The model under review builds one solid part; all positions refer to its coordinate system, in mm. A direction names the side the tool comes from. Give positions to 0.01 mm unless a question says otherwise; leave off trailing zeros. Order: outer loops, then holes, each group sorted by start corner. A loop starts at its lowest first (then second) coordinate and runs counter-clockwise, first axis right, second up. Notation, with made-up numbers: (-12, 72.5) -> (38, 72.5) arc R8 cw to (38, 79.5) -> close; hole circle Ø9 at (26.5, 88.5). An arc over 180 degrees is marked (long way). Answer as a JSON object with one key per item and string values. Group by question number.
from build123d import *

# Parameters (mm, degrees)
F0_R     = 3.5
F0_R_2   = 3
F1_DEPTH = 17.016
F3_R     = 4.5
F3_R_2   = 3.5
F4_DEPTH = 16
F6_W     = 16
F6_H     = 9


with BuildPart() as f1:
    # F0 (on Top) → F1 (new body)
    with BuildSketch(Plane.XY):
        Circle(F0_R)
        Circle(F0_R_2, mode=Mode.SUBTRACT)
    extrude(amount=F1_DEPTH)

    # F3 (on offset) → F4 (join, through all)
    with BuildSketch(Plane.XY.offset(1.016)):
        Circle(F3_R)
        Circle(F3_R_2, mode=Mode.SUBTRACT)
    extrude(amount=F4_DEPTH)

    # F6 (on offset) → F7 section 0
    with BuildSketch(Plane.XY.offset(17.016), mode=Mode.PRIVATE) as f7_s0:
        Rectangle(F6_W, F6_H)
    loft([f7_s0.sketch, Vertex(0, 0, 1.016)], mode=Mode.SUBTRACT)


solid = f1.part
1. Take a section at A-A on x = 0. Give the boundary of the cut face in (y, z).
2. For probe 1 along Y at (x, z) = (0, 3.5); probe 2 along X at (y, z) = (0, 8.75), list the stretches that pass through material, from the lowest coordinate up. Write a range as [from, to].
3. For pin 1 (1.5 mm diameter, centred on x = -2, z = 14.5, fed in from +Y); pin 2 (2 mm diameter, centred on x = -1.5, z = 10.5, fed in from +Y); pin 3 (4 mm diameter, centred on y = -3.5, z = 6.5, fed in from -X), all flat-tipped, find the tip position at first contact; note any pin that passes through.
4. Take a section at D-D on x = 3.25. Give the boundary of the cut face in (y, z), plus the area to 3 significant figures.
5. Take a section at C-C on z = 10.25. Give the boundary of the cut face in (x, y).
6. Machinability: for faces 1 (the flat face through (3, 1, 0)), 2 (the flat face through (3.54, -0.03, 8.1)), 3 (the cylindrical face through (3.233, -1.341, 0.501)), which of the approach directions +Z, -Z, +X, -X, +Y, -Y give a long, thin tool a straight path to every point of the face, cutting with its end or side? Answer none if there is none.
7. Take a section at B-B on y = 0. Give the boundary of the cut face in (x, z).
8. Draft analysis for pull direction X (two halves, no side actions). For faces 4 (the cylindrical face through (4.292, 1.352, 7.126)), 5 (the cylindrical face through (2.86, 0.9, 4.48)), 6 (the flat face through (0, -4, 1.016)), state which applies: pulls with the +X half, pulls with the -X half, needs draft (parallel to the pull), parting line crosses it, or undercut.
Checks:
{
 "1": {"outline": "(-4.5, 1.02) -> (-3.5, 1.02) -> (-3.5, 0) -> (-3, 0) -> (-3, 11.68) -> (-4.5, 17.02) -> close; (3, 0) -> (3.5, 0) -> (3.5, 1.02) -> (4.5, 1.02) -> (4.5, 17.02) -> (3, 11.68) -> close"},
 "2": {"probe 1": "y = [-4.5, -3], [3, 4.5]", "probe 2": "x = [-4.5, -3.87], [3.87, 4.5]"},
 "3": {"pin 1": "stops at y = 4.32", "pin 2": "stops at y = 4.47", "pin 3": "stops at x = -4.24"},
 "4": {"outline": "(-3.11, 1.02) -> (-1.3, 1.02) -> (-1.3, 0) -> (1.3, 0) -> (1.3, 1.02) -> (3.11, 1.02) -> (3.11, 12.08) -> (1.83, 7.52) -> (-1.83, 7.52) -> (-3.11, 12.08) -> close", "area": "49.0 mm2"},
 "5": {"outline": "(-3.67, -2.6) arc R4.5 ccw to (3.67, -2.6) -> (1.5, -2.6) arc R3 cw to (-1.5, -2.6) -> close; (-3.67, 2.6) -> (-1.5, 2.6) arc R3 cw to (1.5, 2.6) -> (3.67, 2.6) arc R4.5 ccw to start"},
 "6": {"face 1": "-Z, +X, -X, +Y, -Y", "face 2": "+Z", "face 3": "-Z"},
 "7": {"outline": "(-4.5, 1.02) -> (-3.5, 1.02) -> (-3.5, 0) -> (-3, 0) -> (-3, 7.02) -> (-4.5, 10.02) -> close; (3, 0) -> (3.5, 0) -> (3.5, 1.02) -> (4.5, 1.02) -> (4.5, 10.02) -> (3, 7.02) -> close"},
 "8": {"face 4": "parting line crosses it", "face 5": "undercut", "face 6": "needs draft"}
}
